```python
from build123d import *

# Parameters (mm, degrees)
F1_DEPTH  = 240
F2_DEPTH  = 5
F5_DEPTH  = 260
F6_DEPTH  = 252
F8_DEPTH  = 5
F10_DEPTH = 5


with BuildPart() as f1:
    # F0 (on Front) → F1 (new body)
    with BuildSketch(Plane.XZ):
        with BuildLine():
            Line((-91.99476, 48.640542), (-111.663712, 48.640542))
            Line((-111.663712, 48.640542), (-111.663712, -61.359458))
            Line((-111.663712, -61.359458), (-36.663712, -61.359458))
            ThreePointArc((-36.663712, -61.359458), (-33.128178, -59.894992), (-31.663712, -56.359458))
            Line((-31.663712, -56.359458), (-31.663712, 0.890209))
            ThreePointArc((-31.663712, 0.890209), (-33.128178, 4.425743), (-36.663712, 5.890209))
            Line((-36.663712, 5.890209), (-48.030325, 5.890209))
            Line((-48.030325, 5.890209), (-48.030325, -12.867237))
            Line((-48.030325, -12.867237), (-64.685345, -18.742749))
            Line((-64.685345, -18.742749), (-87.279566, 45.303955))
            ThreePointArc((-87.279566, 45.303955), (-89.106601, 47.722028), (-91.99476, 48.640542))
        make_face()
    extrude(amount=F1_DEPTH)

    # F0 (on Front) → F2 (join)
    with BuildSketch(Plane.XZ):
        Polygon((-48.030325, 5.890209), (-87.279566, 45.303955), (-64.685345, -18.742749), (-48.030325, -12.867237), align=None)
    extrude(amount=F2_DEPTH)

    # F4 (on face) → F5 (cut)
    with BuildSketch(Plane.XZ.offset(240)):
        Polygon((-91.99476, 43.640542), (-106.663712, 43.640542), (-106.663712, -56.359458), (-67.737126, -56.359458), (-67.737126, -25.121357), align=None)
    extrude(amount=-F5_DEPTH, mode=Mode.SUBTRACT)

    # F3 (on face) → F6 (cut)
    with BuildSketch(Plane.XZ.offset(240)):
        Polygon((-47.102027, -18.742749), (-62.739263, -24.259211), (-57.695907, -38.493532), (-42.078068, -32.983914), align=None)
    extrude(amount=-F6_DEPTH, mode=Mode.SUBTRACT)

    # F7 (on face) → F8 (join)
    with BuildSketch(Plane.XZ.offset(240)):
        Polygon((-48.030325, -12.867237), (-48.030325, 5.890209), (-87.279566, 45.303955), (-64.685345, -18.742749), align=None)
    extrude(amount=-F8_DEPTH)

    # F9 (on face) → F10 (cut)
    with BuildSketch(Plane(origin=(-111.663712, 0, 0), x_dir=(0, -1, 0), z_dir=(-1, 0, 0))):
        Polygon((227.999998, -49.359457), (227.999998, 36.64054), (12.000002, 36.64054), (12.000002, 5.890209), (12.000002, 0.890209), (12.000002, -49.359457), align=None)
    extrude(amount=-F10_DEPTH, mode=Mode.SUBTRACT)


solid = f1.part
```
Geometry check sheet. Reference: the model listing, model coordinates, mm. A direction names the side the tool comes from. Give positions to 0.01 mm unless a question says otherwise; leave off trailing zeros. Write each loop counter-clockwise with the first axis right and the second up, starting at its lowest first coordinate (ties: lowest second). Pieces come first, ordered by that corner, then holes.
1) Section check C-C, the plane y = -200.5. Record the boundary of the cut face in (x, z), and give its area (3 significant figures).
2) Section check A-A, the plane z = -42.5. Record the boundary of the cut face in (x, y), and give its area (3 significant figures).
3) Section check B-B, the plane z = -54. Record the boundary of the cut face in (x, y).
4) Material ranges on L1, parallel to Z at x = -93, y = -115.5; L2, parallel to X at y = -209, z = -54; L3, parallel to Y at x = -54, z = -8.5, recorded low to high.
5) Release check for a two-part mould opening along Z. For faces 1 (the flat face through (-109, -122, 36.641)), 2 (the flat face through (-56.241, -118.39, -15.764)), 3 (the flat face through (-50, -121.68, -35.78)), 4 (the cylindrical face through (-33.167, -118.32, -59.934)) record: pulls with the +Z half, pulls with the -Z half, needs draft (parallel to the pull), parting line crosses it, or undercut.
6) Gauge pin test, flat ends, axial feed: pin 1 (2 mm diameter, centred on y = -198, z = 34, fed in from -X); pin 2 (3.5 mm diameter, centred on x = -43, y = -71, fed in from +Z); pin 3 (3 mm diameter, centred on y = -39, z = 24.5, fed in from +X); pin 4 (5.5 mm diameter, centred on x = -109, z = -17, fed in from +Y). Record the tip position at first contact, or that the pin passes through.
7) Section check D-D, the plane z = -16. Record the boundary of the cut face in (x, y).
8) Access from +Z, -Z, +X, -X, +Y, -Y to the whole of each face (thin tool, end or side, straight path). Record for faces 5 (the flat face through (-54.81, -121.68, -21.46)), 6 (the flat face through (-42, -118, 5.89)), 7 (the flat face through (-48.03, -118, -3)), 8 (the flat face through (-109, -118, -49.359)).
Computed:
1. outline: (-111.66, -61.36) - (-36.66, -61.36) arc R5 ccw to (-31.66, -56.36) - (-31.66, 0.89) arc R5 ccw to (-36.66, 5.89) - (-48.03, 5.89) - (-48.03, -12.87) - (-64.69, -18.74) - (-87.28, 45.3) arc R5 ccw to (-91.99, 48.64) - (-111.66, 48.64) - (-111.66, 36.64) - (-106.66, 36.64) - (-106.66, 43.64) - (-91.99, 43.64) - (-67.74, -25.12) - (-67.74, -56.36) - (-106.66, -56.36) - (-106.66, -49.36) - (-111.66, -49.36) - close; hole (-62.74, -24.26) - (-57.7, -38.49) - (-42.08, -32.98) - (-47.1, -18.74) - close
1. area: 2,470 mm2
2. outline: (-111.66, -240) - (-106.66, -240) - (-106.66, -228) - (-111.66, -228) - close; (-111.66, -12) - (-106.66, -12) - (-106.66, 0) - (-111.66, 0) - close; (-67.74, -240) - (-31.66, -240) - (-31.66, 0) - (-67.74, 0) - close
2. area: 8,780 mm2
3. outline: (-111.66, -240) - (-106.66, -240) - (-106.66, 0) - (-111.66, 0) - close; (-67.74, -240) - (-31.66, -240) - (-31.66, 0) - (-67.74, 0) - close
4. L1: z = -61.36 to -56.36, 43.64 to 48.64
4. L2: x = -111.66 to -106.66, -67.74 to -31.66
4. L3: y = -240 to -235, -5 to 0
5. face 1: undercut
5. face 2: pulls with the +Z half
5. face 3: undercut
5. face 4: pulls with the -Z half
6. pin 1: stops at x = -88.95
6. pin 2: stops at z = 5.89
6. pin 3: stops at x = -79.41
6. pin 4: stops at y = 0
7. outline: (-111.66, -240) - (-106.66, -240) - (-106.66, -228) - (-111.66, -228) - close; (-111.66, -12) - (-106.66, -12) - (-106.66, 0) - (-111.66, 0) - close; (-70.95, -240) - (-31.66, -240) - (-31.66, 0) - (-70.95, 0) - close; hole (-65.65, -235) - (-56.91, -235) - (-56.91, -5) - (-65.65, -5) - close
8. face 5: +Y, -Y
8. face 6: +Z, +X, +Y, -Y
8. face 7: +Z
8. face 8: -X
